Check sheet for the modelled part. Datum: model origin and axes. Units: mm. Round coordinates to 2 decimals unless told otherwise and drop trailing zeros. Write each loop counter-clockwise with the first axis right and the second up, starting at its lowest first coordinate (ties: lowest second). Pieces come first, ordered by that corner, then holes. Notation, with made-up numbers: (-24.5, 67) -> (-8.5, 67) arc R33 ccw to (-8.5, 104) -> close; hole circle Ø3 at (88.25, -36.75). An arc over 180 degrees is marked (long way). Put each result on its own line as item: value. Start each with the question number.
from build123d import *

# Parameters (mm, degrees)
F1_DEPTH = 3.175


with BuildPart() as f1:
    # F0 (on Front) → F1 (new body)
    with BuildSketch(Plane.XZ):
        with BuildLine():
            Line((-25.0390999136, 10.2285252111), (-37.7390999136, 10.2285252111))
            Line((-37.7390999136, 10.2285252111), (-37.7390999136, -2.4714747889))
            Line((-37.7390999136, -2.4714747889), (-34.9609749136, -2.4714747889))
            ThreePointArc((-34.9609749136, -2.4714747889), (-33.2835837944, 0.7689960166), (-29.6693082469, 1.2702985949))
            ThreePointArc((-29.6693082469, 1.2702985949), (-27.6046848946, 2.90044023), (-25.0390999136, 3.4816502111))
            Line((-25.0390999136, 3.4816502111), (-25.0390999136, 10.2285252111))
        make_face()
        with BuildLine():
            Line((-12.3390999136, 10.2285252111), (-25.0390999136, 10.2285252111))
            Line((-25.0390999136, 10.2285252111), (-25.0390999136, 3.4816502111))
            ThreePointArc((-25.0390999136, 3.4816502111), (-20.8296048568, 1.7380202678), (-19.0859749136, -2.4714747889))
            Line((-19.0859749136, -2.4714747889), (-12.3390999136, -2.4714747889))
            Line((-12.3390999136, -2.4714747889), (-12.3390999136, 10.2285252111))
        make_face()
        with BuildLine():
            Line((-12.3390999136, -15.1714747889), (-12.3390999136, -2.4714747889))
            Line((-12.3390999136, -2.4714747889), (-19.0859749136, -2.4714747889))
            ThreePointArc((-19.0859749136, -2.4714747889), (-20.8296048568, -6.6809698457), (-25.0390999136, -8.4245997889))
            Line((-25.0390999136, -8.4245997889), (-25.0390999136, -15.1714747889))
            Line((-25.0390999136, -15.1714747889), (-12.3390999136, -15.1714747889))
        make_face()
        with BuildLine():
            Line((-34.9609749136, -2.4714747889), (-37.7390999136, -2.4714747889))
            Line((-37.7390999136, -2.4714747889), (-37.7390999136, -15.1714747889))
            Line((-37.7390999136, -15.1714747889), (-25.0390999136, -15.1714747889))
            Line((-25.0390999136, -15.1714747889), (-25.0390999136, -8.4245997889))
            ThreePointArc((-25.0390999136, -8.4245997889), (-27.6046848946, -7.8433898078), (-29.6693082469, -6.2132481727))
            ThreePointArc((-29.6693082469, -6.2132481727), (-33.2835837944, -5.7119455945), (-34.9609749136, -2.4714747889))
        make_face()
    extrude(amount=F1_DEPTH)


solid = f1.part
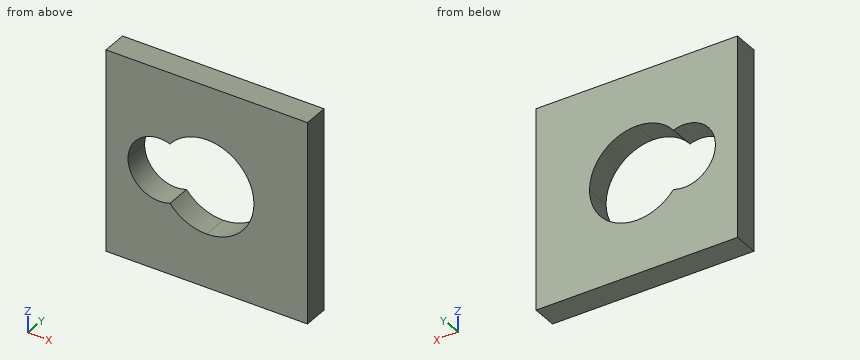
1. Section check C-C, the plane x = -27.5. Enter the section's corners in (y, z) (3 decimals).
2. Section check A-A, the plane x = -31. Enter the section's corners in (y, z) (3 decimals).
3. Section check B-B, the plane y = -1.95. Enter the section's corners in (x, z).
4. Material ranges on L1, parallel to Z at x = -32.5, y = -2.75; L2, parallel to X at y = -0.9, z = -5.5; L3, parallel to Z at x = -23, y = -0.35, recorded low to high. Write a range as [from, to].
5. Gauge pin test, flat end, axial feed: P1, Ø1, axis at x = -25, z = 3.5, coming from the +Y side. Record the tip position at first contact, or that the pin passes through.
Reply:
1. outline: (-3.175, -15.171) -> (0, -15.171) -> (0, -7.892) -> (-3.175, -7.892) -> close; (-3.175, 2.949) -> (0, 2.949) -> (0, 10.229) -> (-3.175, 10.229) -> close
2. outline: (-3.175, -15.171) -> (0, -15.171) -> (0, -6.44) -> (-3.175, -6.44) -> close; (-3.175, 1.497) -> (0, 1.497) -> (0, 10.229) -> (-3.175, 10.229) -> close
3. outline: (-37.74, -15.17) -> (-12.34, -15.17) -> (-12.34, 10.23) -> (-37.74, 10.23) -> close; hole (-29.67, -6.21) arc R5.95 ccw (long way) to (-29.67, 1.27) arc R3.97 ccw (long way) to start
4. L1: z = [-15.17, -6.14], [1.2, 10.23]
4. L2: x = [-37.74, -33.56], [-19.91, -12.34]
4. L3: z = [-15.17, -8.06], [3.12, 10.23]
5. P1: stops at y = 0
